Here's the drawing with two shaded views (mm, measured from the low corner). I have some questions. Round coordinates to 2 decimals unless told otherwise and drop trailing zeros. Loops run counter-clockwise (first coordinate to the right, second up) from the corner with the lowest first, then second, coordinate; pieces in that order, holes last. Notation, with made-up numbers: (-25, 67.5) -> (-1, 67.5) arc R19 cw to (-1, 86.5) -> close; hole circle Ø11 at (53.25, -16). An arc over 180 degrees is marked (long way). Write item = value, one per line.
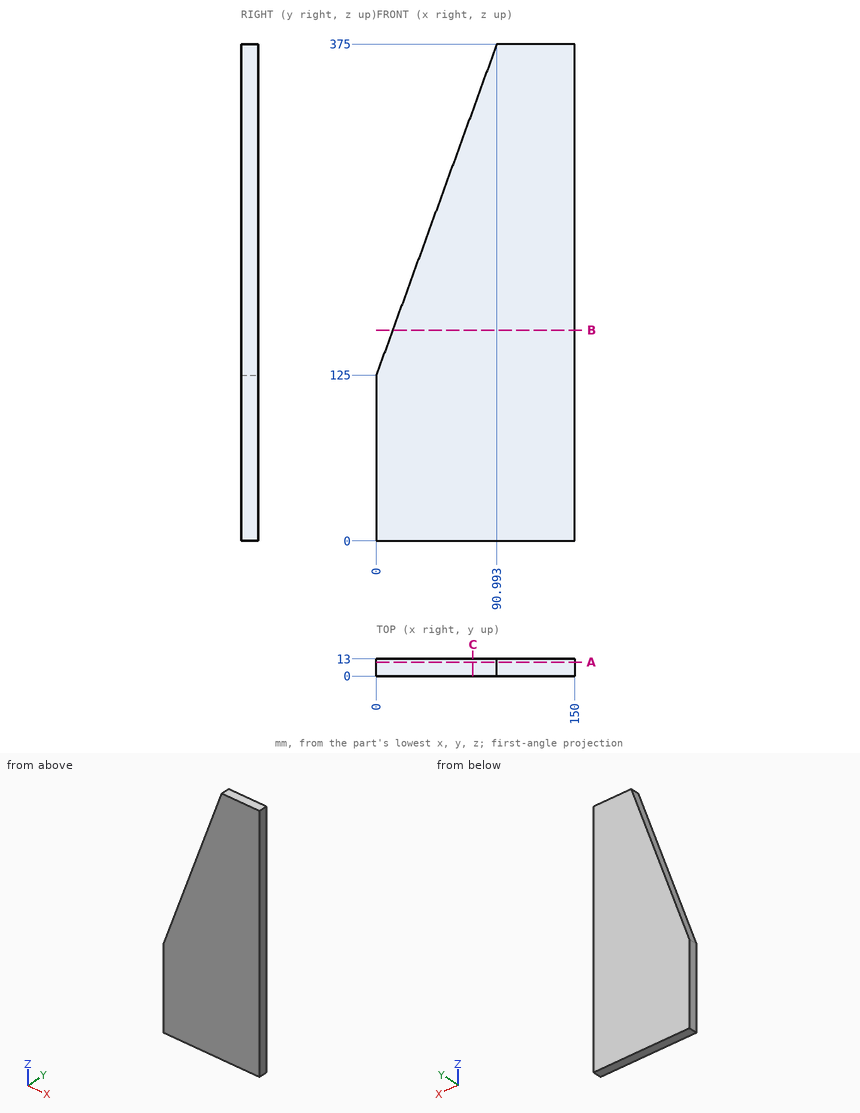
1. Suppose I cut it at B-B, the plane z = 159. List the corners of the cut face in (x, y) for me (1 decimal), and give its area (3 significant figures).
Entries:
outline = (12.4, 0) -> (150, 0) -> (150, 13) -> (12.4, 13) -> close
area = 1,790 mm²
2. I'm going to push a flat-ended pin straight in: pin 1 (4 mm diameter, centred on y = 4, z = 313, fed in from -X). Where does the tip first touch, or does it pass through?
Entries:
pin_1 = 67.7
3. Suppose I cut it at C-C, the plane x = 73. List the corners of the cut face in (y, z) for me (1 decimal).
Entries:
outline = (0, 0) -> (13, 0) -> (13, 325.6) -> (0, 325.6) -> close
4. I need wall thicknesses on line 1 (X direction, y = 9.25, z = 305.5); line 2 (X direction, y = 6, z = 139.5). Which ranges of each line are inside material? Lowest first, please. Write a range as [from, to].
Entries:
line_1 = [65.7, 150]
line_2 = [5.28, 150]
5. Suppose I cut it at A-A, the plane y = 10.5. List the corners of the cut face in (x, z) for me.
Entries:
outline = (0, 0) -> (150, 0) -> (150, 375) -> (90.99, 375) -> (0, 125) -> close
